The figure shows three views and two pictorial views of one solid part (mm, origin at its lowest corner). Answer the questions. A direction names the side the tool comes from. Give positions to 0.01 mm unless a question says otherwise; leave off trailing zeros. Order: outer loops, then holes, each group sorted by start corner. A loop starts at its lowest first (then second) coordinate and runs counter-clockwise, first axis right, second up. Notation, with made-up numbers: (63.25, 45.25) - (109.25, 45.25) arc R37 ccw to (109.25, 83.25) - close; hole circle Ø3 at (18.5, -21.5). An arc over 180 degrees is marked (long way). Answer as a JSON object with one key per item and string values. Group by question number.
Q1. Consider line 1 (X direction, y = 229, z = 5.5); line 2 (Y direction, x = 81.5, z = 15.5). Determine where each line is inside the solid, lowest interval first.
Q2. For the marked faces 1 and 2, determine the directions among +Z, -Z, +X, -X, +Y, -Y from which every point of the face is accessible in a straight line to the end or side of a thin tool.
Q3. A cutting plane is placed at C-C, the plane x = 33.5. Give the vertices of the cut face in (y, z), and give its area (3 significant figures).
Q4. A cutting plane is placed at B-B, the plane z = 16.75. Give the vertices of the cut face in (x, y), and give its area (3 significant figures).
Q5. A cutting plane is placed at A-A, the plane y = 75. Give the vertices of the cut face in (x, z).
Q6. Given pin 1 (1.5 mm diameter, centred on x = 14.5, z = 12.5, fed in from -Y); pin 2 (1 mm diameter, centred on y = 110, z = 6.5, fed in from -X), each flat-ended and moving along its own axis, determine where each tip first touches the part or whether it passes through.
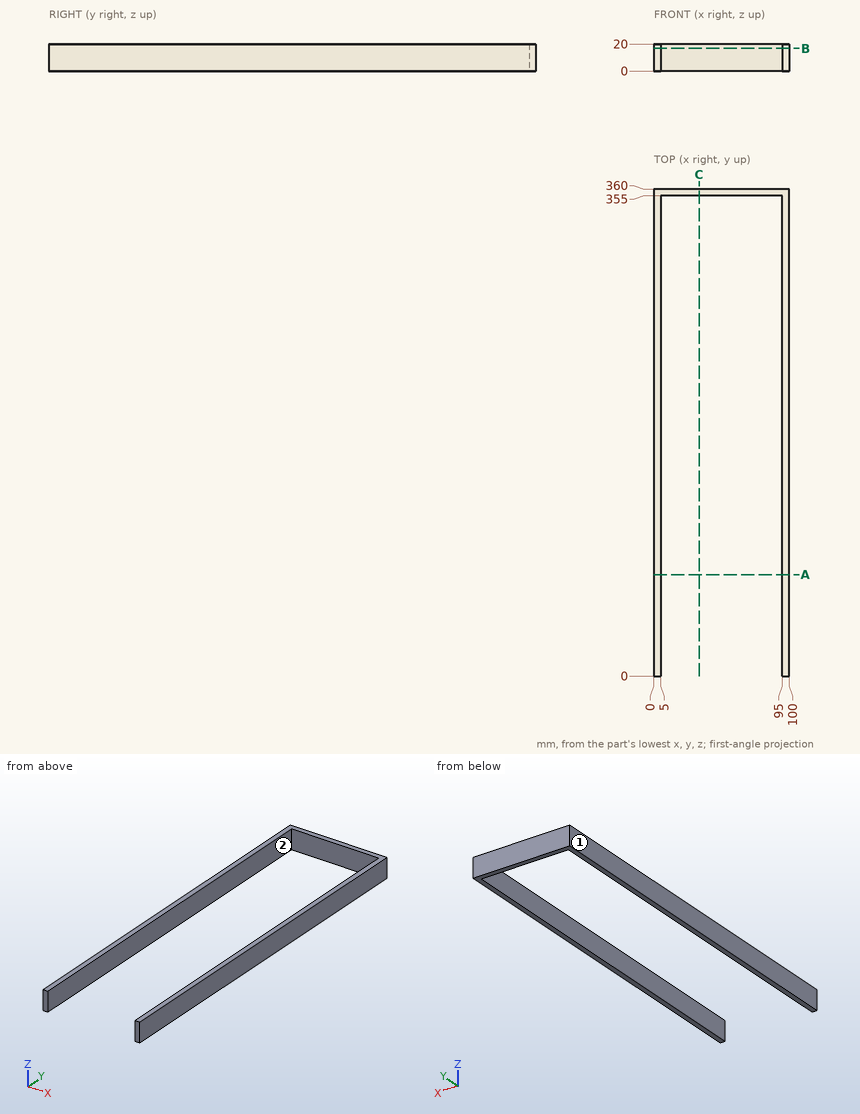
Reply:
{
 "1": {"line 1": "x = 0 to 5, 95 to 100", "line 2": "y = 355 to 360"},
 "2": {"face 1": "+Z, -Z, -X, +Y, -Y", "face 2": "+Z, -Z, -Y"},
 "3": {"outline": "(355, 0) - (360, 0) - (360, 20) - (355, 20) - close", "area": "100 mm^2"},
 "4": {"outline": "(0, 0) - (5, 0) - (5, 355) - (95, 355) - (95, 0) - (100, 0) - (100, 360) - (0, 360) - close", "area": "4,050 mm^2"},
 "5": {"outline": "(0, 0) - (5, 0) - (5, 20) - (0, 20) - close; (95, 0) - (100, 0) - (100, 20) - (95, 20) - close"},
 "6": {"pin 1": "stops at y = 355", "pin 2": "stops at x = 0"}
}
